from build123d import *

# Parameters (mm, degrees)
SKETCH184_W          = 20
SKETCH184_H          = 40
PAD049_DEPTH         = 40
SKETCH185_R          = 1.55
POCKET100_DEPTH      = 6
SKETCH186_R          = 1.55
POCKET101_DEPTH      = 6
SKETCH187_R          = 1.55
POCKET102_DEPTH      = 8
SKETCH188_R          = 2.55
POCKET103_DEPTH      = 20
SKETCH189_R          = 2.55
POCKET104_DEPTH      = 14
POCKET105_DEPTH      = 5.5
SKETCH191_R          = 1.55
POCKET106_DEPTH      = 53.206
POCKET106_DEPTH_BACK = 53.206
SKETCH192_R          = 3
POCKET107_DEPTH      = 31.206
SKETCH193_R          = 3
POCKET108_DEPTH      = 31.206
FILLET047_R          = 2


with BuildPart() as part:
    # Sketch184 → Pad049 (new body)
    with BuildSketch(Plane.XY):
        with BuildLine():
            Line((-53.205, 0), (-16.535, 63.5143031136))
            Line((-16.535, 63.5143031136), (-33.8555080757, 73.5143031136))
            Line((-33.8555080757, 73.5143031136), (-21.7278633238, 94.52))
            ThreePointArc((-13.0676092859, 99.52), (-18.0676092859, 98.1802540378), (-21.7278633238, 94.52))
            Line((-13.0676092859, 99.52), (13.0676092859, 99.52))
            ThreePointArc((21.7278633238, 94.52), (18.0676092859, 98.1802540378), (13.0676092859, 99.52))
            Line((33.8555080757, 73.5143031136), (21.7278633238, 94.52))
            Line((16.535, 63.5143031136), (33.8555080757, 73.5143031136))
            Line((53.205, 0), (16.535, 63.5143031136))
            Line((53.205, 0), (48.0088475773, -3))
            Line((48.0088475773, -3), (40.9247597743, 9.27))
            ThreePointArc((40.9247597743, 9.27), (39.0946327554, 11.1001270189), (36.5946327554, 11.77))
            Line((-36.5946327554, 11.77), (36.5946327554, 11.77))
            ThreePointArc((-36.5946327554, 11.77), (-39.0946327554, 11.1001270189), (-40.9247597743, 9.27))
            Line((-48.0088475773, -3), (-40.9247597743, 9.27))
            Line((-53.205, 0), (-48.0088475773, -3))
        make_face()
        with Locations((0, 73.52)):
            Rectangle(SKETCH184_W, SKETCH184_H, mode=Mode.SUBTRACT)
        with BuildLine():
            Line((-27.3570284484, 32.77), (-34.2852316787, 20.77))
            ThreePointArc((-34.2852316787, 20.77), (-34.2852316787, 18.77), (-32.5531808711, 17.77))
            Line((-32.5531808711, 17.77), (32.5531808711, 17.77))
            ThreePointArc((32.5531808711, 17.77), (34.2852316787, 18.77), (34.2852316787, 20.77))
            Line((34.2852316787, 20.77), (27.3570284484, 32.77))
            ThreePointArc((27.3570284484, 32.77), (24.4288252181, 35.6982032303), (20.4288252181, 36.77))
            Line((20.4288252181, 36.77), (-20.4288252181, 36.77))
            ThreePointArc((-20.4288252181, 36.77), (-24.4288252181, 35.6982032303), (-27.3570284484, 32.77))
        make_face(mode=Mode.SUBTRACT)
    extrude(amount=PAD049_DEPTH)

    # Sketch185 (on DatumPlane) → Pocket100 (cut, symmetric)
    with BuildSketch(Plane(origin=(53, 0, 0), x_dir=(-0.5, 0.8660254038, 0), z_dir=(0.8660254038, 0.5, 0))):
        with Locations((47.2375, 30)):
            Circle(SKETCH185_R)
        with Locations((9.8975, 30)):
            Circle(SKETCH185_R)
        with Locations((47.2375, 10)):
            Circle(SKETCH185_R)
        with Locations((9.8975, 10)):
            Circle(SKETCH185_R)
    extrude(amount=POCKET100_DEPTH, both=True, mode=Mode.SUBTRACT)

    # Sketch186 (on DatumPlane) → Pocket101 (cut, symmetric)
    with BuildSketch(Plane(origin=(-53, 0, 0), x_dir=(0.5, 0.8660254038, 0), z_dir=(0.8660254038, -0.5, 0))):
        with Locations((47.2375, 30)):
            Circle(SKETCH186_R)
        with Locations((47.2375, 10)):
            Circle(SKETCH186_R)
        with Locations((9.8975, 10)):
            Circle(SKETCH186_R)
        with Locations((9.8975, 30)):
            Circle(SKETCH186_R)
    extrude(amount=POCKET101_DEPTH, both=True, mode=Mode.SUBTRACT)

    # Sketch187 → Pocket102 (cut)
    with BuildSketch(Plane(origin=(0, 99.52, 0), x_dir=(-1, 0, 0), z_dir=(0, 1, 0))):
        with Locations((0, 30)):
            Circle(SKETCH187_R)
        with Locations((0, 10)):
            Circle(SKETCH187_R)
    extrude(amount=-POCKET102_DEPTH, mode=Mode.SUBTRACT)

    # Sketch188 → Pocket103 (cut)
    with BuildSketch(Plane.XZ):
        with Locations((0, 20)):
            Circle(SKETCH188_R)
    extrude(amount=-POCKET103_DEPTH, mode=Mode.SUBTRACT)

    # Sketch189 → Pocket104 (cut)
    with BuildSketch(Plane.XZ.offset(-53.52)):
        with Locations((0, 20)):
            Circle(SKETCH189_R)
    extrude(amount=POCKET104_DEPTH, mode=Mode.SUBTRACT)

    # Sketch190 → Pocket105 (cut)
    with BuildSketch(Plane.XZ.offset(-53.52)):
        Polygon((4.1, 17.6328638963), (4.1, 22.3671361037), (0, 24.7342722074), (-4.1, 22.3671361037), (-4.1, 17.6328638963), (0, 15.2657277926), align=None)
    extrude(amount=POCKET105_DEPTH, mode=Mode.SUBTRACT)

    # Sketch191 → Pocket106 (cut, two sides)
    with BuildSketch(Plane.YZ) as pocket106_sk:
        with Locations((83.52, 30)):
            Circle(SKETCH191_R)
        with Locations((83.52, 10)):
            Circle(SKETCH191_R)
    extrude(amount=-POCKET106_DEPTH, mode=Mode.SUBTRACT)
    extrude(pocket106_sk.sketch, amount=POCKET106_DEPTH_BACK, mode=Mode.SUBTRACT)

    # Sketch192 → Pocket107 (cut, through all)
    with BuildSketch(Plane.YZ.offset(22)):
        with Locations((83.52, 30)):
            Circle(SKETCH192_R)
        with Locations((83.52, 10)):
            Circle(SKETCH192_R)
    extrude(amount=POCKET107_DEPTH, mode=Mode.SUBTRACT)

    # Sketch193 → Pocket108 (cut, through all)
    with BuildSketch(Plane.YZ.offset(-22)):
        with Locations((83.52, 30)):
            Circle(SKETCH193_R)
        with Locations((83.52, 10)):
            Circle(SKETCH193_R)
    extrude(amount=-POCKET108_DEPTH, mode=Mode.SUBTRACT)

    # Fillet047
    fillet047_edges = [part.edges().sort_by_distance(p)[0] for p in [
        (27.791686, 84.017152, 40),
        (18.067609, 98.180254, 40),
        (0, 99.52, 40),
        (-18.067609, 98.180254, 40),
        (-27.791686, 84.017152, 40),
        (27.791686, 84.017152, 0),
        (18.067609, 98.180254, 0),
        (0, 99.52, 0),
        (-18.067609, 98.180254, 0),
        (-27.791686, 84.017152, 0),
    ]]
    fillet(fillet047_edges, radius=FILLET047_R)


solid = part.part
Input: part model. Units: mm. Frame: model coordinates. A direction names the side the tool comes from. Coordinates: 2 decimals unless noted, no trailing zeros. Loops run counter-clockwise (first coordinate to the right, second up) from the corner with the lowest first, then second, coordinate; pieces in that order, holes last.
(1) Section C-C on z = 10. Count the separate pieces of the cut face and the enclosed holes in it, then the cut area to 3 significant figures.
(2) Set-up query: faces 4 (the face through (44.516, 3.049, 19.72)), 5 (the face through (1.18, 14.73, 17.74)), 6 (the face through (25.045, 80.523, 10.132)), 7 (the face through (30.87, 26.686, 19.72)), 8 (the face through (-25.045, 80.523, 10.132)). Return all of +Z, -Z, +X, -X, +Y, -Y with unobstructed straight access to the full face (end or side cutting, diameter ignored); none if empty.
(3) Pull-direction query (X, two-part tool) for faces 1 (the face through (0, 39.52, 20)), 2 (the face through (15.916, 84.998, 30.466)), 3 (the face through (35.13, 31.31, 19.72)); classes: released by +X, released by -X, zero draft, split by the parting line, or undercut.
(4) Section B-B on y = 51. Return the cut outline in (x, z).
(5) Material intervals for probe 1 along Z at (x, y) = (-14, 83.52); probe 2 along Y at (x, z) = (-1, 36.5); probe 3 along Y at (x, z) = (13.5, 10), sorted ascending.
(6) First-contact query: pin 1 Ø1.4 at (y, z) = (51.5, 19.5) entering from -X; pin 2 Ø5.5 at (y, z) = (83.52, 10) entering from +X; pin 3 Ø7 at (y, z) = (83.52, 30) entering from -X; pin 4 Ø4 at (x, y) = (-39, 32.5) entering from -Z. Flat tips, straight axial feed; report the tip coordinate or a pass-through.
(7) Section A-A on y = 26.5. Return the cut outline in (x, z).
Data:
1. separate pieces: 5
1. enclosed holes: 1
1. area: 3,120 mm2
2. face 4: +Z, -Z, -Y
2. face 5: -Y
2. face 6: +X
2. face 7: +Z, -Z
2. face 8: -X
3. face 1: undercut
3. face 2: zero draft
3. face 3: released by +X
4. outline: (-23.76, 0) - (23.76, 0) - (23.76, 40) - (-23.76, 40) - close; hole (-4.1, 17.63) - (0, 15.27) - (4.1, 17.63) - (4.1, 22.37) - (0, 24.73) - (-4.1, 22.37) - close
5. probe 1: z = 0 to 8.45, 11.55 to 28.45, 31.55 to 40
5. probe 2: y = 11.77 to 17.77, 36.77 to 53.52, 93.52 to 99.52
5. probe 3: y = 11.77 to 17.77, 36.77 to 81.97, 85.07 to 99.51
6. pin 1: stops at x = -23.88
6. pin 2: stops at x = 22
6. pin 3: stops at x = -30.1
6. pin 4: passes through
7. outline: (-37.91, 0) - (-30.98, 0) - (-30.98, 40) - (-37.91, 40) - close; (30.98, 0) - (37.91, 0) - (37.91, 40) - (30.98, 40) - close
